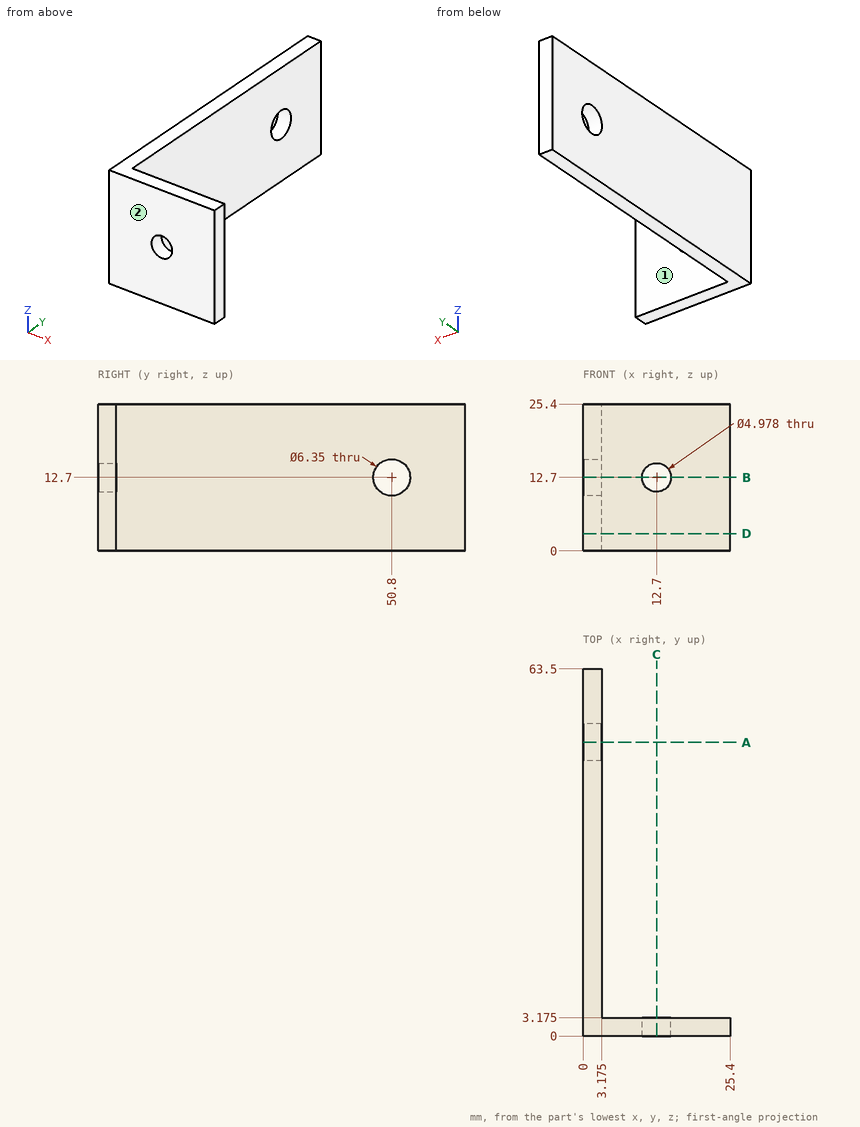
Geometry check sheet. Reference: drawing and pictorial views, mm from the part's lowest x, y, z. A direction names the side the tool comes from. Coordinates: 2 decimals unless noted, no trailing zeros. Order: outer loops, then holes, each group sorted by start corner. A loop starts at its lowest first (then second) coordinate and runs counter-clockwise, first axis right, second up. Notation, with made-up numbers: M 65,2 L 113,2 A20 cw 113,22 Z; hole C 68.25,-15.75 d2. An arc over 180 degrees is marked long. Return JSON: item names as keys, results as strings.
1) Access from +Z, -Z, +X, -X, +Y, -Y to the whole of each face (thin tool, end or side, straight path). Record for the marked faces 1 and 2.
Answer list:
{"face 1": "+Z, -Z, +X, +Y", "face 2": "+Z, -Z, +X, -X, -Y"}
2) Gauge pin test, flat ends, axial feed: pin 1 (12 mm diameter, centred on y = 39.5, z = 13.5, fed in from +X) (3 decimals); pin 2 (1.5 mm diameter, centred on x = 4.5, y = 52.5, fed in from +Z); pin 3 (6 mm diameter, centred on x = 11, z = 9.5, fed in from +Y) (3 decimals). Record the tip position at first contact, or that the pin passes through.
Answer list:
{"pin 1": "x = 3.175", "pin 2": "through", "pin 3": "y = 3.175"}
3) Cross-section at B-B, the plane z = 12.7. Record the boundary of the cut face in (x, y) (1 decimal), and give its area (3 significant figures).
Answer list:
{"outline": "M 0,0 L 10.2,0 L 10.2,3.2 L 3.2,3.2 L 3.2,47.6 L 0,47.6 Z; M 0,54 L 3.2,54 L 3.2,63.5 L 0,63.5 Z; M 15.2,0 L 25.4,0 L 25.4,3.2 L 15.2,3.2 Z", "area": "236 mm2"}
4) Cross-section at D-D, the plane z = 3. Record the boundary of the cut face in (x, y) (1 decimal), and give its area (3 significant figures).
Answer list:
{"outline": "M 0,0 L 25.4,0 L 25.4,3.2 L 3.2,3.2 L 3.2,63.5 L 0,63.5 Z", "area": "272 mm2"}
5) Thickness scan on L1, parallel to X at y = 2.45, z = 12.7; L2, parallel to Y at x = 0.7, z = 12.7 (1 decimal). Record the ranges inside material, lowest first. Write a range as [from, to].
Answer list:
{"L1": "[0, 10.21], [15.19, 25.4]", "L2": "[0, 47.6], [54, 63.5]"}
6) Cross-section at A-A, the plane y = 50.8. Record the boundary of the cut face in (x, z) (1 decimal).
Answer list:
{"outline": "M 0,0 L 3.2,0 L 3.2,9.5 L 0,9.5 Z; M 0,15.9 L 3.2,15.9 L 3.2,25.4 L 0,25.4 Z"}
7) Cross-section at C-C, the plane x = 12.7. Record the boundary of the cut face in (y, z) (1 decimal).
Answer list:
{"outline": "M 0,0 L 3.2,0 L 3.2,10.2 L 0,10.2 Z; M 0,15.2 L 3.2,15.2 L 3.2,25.4 L 0,25.4 Z"}
